from build123d import *

# Parameters (mm, degrees)
EXTRUDE_1_DEPTH     = 44
SKETCH_2_OUTSIDE_W  = 114.91
SKETCH_2_OUTSIDE_H  = 31.91
CUT_EXTRUDE_1_DEPTH = 44
SKETCH_3_W          = 83
SKETCH_3_H          = 84.111264856
CUT_EXTRUDE_2_DEPTH = 2
SKETCH_5_W          = 50
SKETCH_5_H          = 50
CUT_EXTRUDE_3_DEPTH = 6
FILLET_1_R          = 40


with BuildPart() as part:
    # Эскиз1 → Бобышка-Вытянуть1 (new body, symmetric)
    with BuildSketch(Plane(origin=(0, 0, 0), x_dir=(0, 0, -1), z_dir=(1, 0, 0))):
        Polygon((44, 0), (-44, 0), (-44, 3), (-25, 5), (25, 5), (44, 3), align=None)
    extrude(amount=EXTRUDE_1_DEPTH, both=True)

    # Эскиз2 outside → Вырез-Вытянуть1 (cut, symmetric)
    with BuildSketch(Plane.XY):
        with Locations((0, 2.5)):
            Rectangle(SKETCH_2_OUTSIDE_W, SKETCH_2_OUTSIDE_H)
        Polygon((44, 0), (-44, 0), (-44, 3), (-25, 5), (25, 5), (44, 3), align=None, mode=Mode.SUBTRACT)
    extrude(amount=CUT_EXTRUDE_1_DEPTH, both=True, mode=Mode.SUBTRACT)

    # Эскиз3 → Вырез-Вытянуть2 (cut)
    with BuildSketch(Plane.XZ):
        Rectangle(SKETCH_3_W, SKETCH_3_H)
    extrude(amount=-CUT_EXTRUDE_2_DEPTH, mode=Mode.SUBTRACT)

    # Эскиз5 → Вырез-Вытянуть3 (cut, through all)
    with BuildSketch(Plane.XZ):
        Rectangle(SKETCH_5_W, SKETCH_5_H)
    extrude(amount=-CUT_EXTRUDE_3_DEPTH, mode=Mode.SUBTRACT)

    # Скругление1
    fillet_1_edges = [part.edges().sort_by_distance(p)[0] for p in [
        (34.5, 4, -34.5),
        (-34.5, 4, -34.5),
        (-34.5, 4, 34.5),
        (34.5, 4, 34.5),
    ]]
    fillet(fillet_1_edges, radius=FILLET_1_R)


solid = part.part
For this review, take the finished solid that the model builds, in its own axes (mm). A direction names the side the tool comes from. Round coordinates to 2 decimals unless told otherwise and drop trailing zeros. Loops run counter-clockwise (first coordinate to the right, second up) from the corner with the lowest first, then second, coordinate; pieces in that order, holes last. Notation, with made-up numbers: (-19, 67) - (-13, 67) arc R30 ccw to (-13, 102) - close; hole circle Ø5 at (-32, 83). An arc over 180 degrees is marked (long way). One line per item, written item: value. Start each with the question number.
Item 1: Take a section at A-A (x = -1). Give the boundary of the cut face in (y, z), plus the area to 3 significant figures.
Item 2: Clearance check with flat-ended pins moving along their axes: pin 1 Ø8 at (x, z) = (-26, -8) entering from -Y; pin 2 Ø12 at (x, z) = (8, -32) entering from +Y. State where each tip first meets the part, or that it passes through.
Item 3: For L1, parallel to Z at x = 22, y = 2.15; L2, parallel to Z at x = -15.5, y = 1.65, list the stretches that pass through material, from the lowest coordinate up.
Item 4: The part is to be moulded in two halves that separate along X. For faces 1 (the flat face through (-44, 2, -1)), 2 (the flat face through (41.5, 1, -1)), 3 (the flat face through (0.56, 3.79, -36.48)), say which applies: +X half, -X half, draft (parallel to the pull), parting line (faces both ways), or undercut.
Item 5: Take a section at B-B (z = -17.5). Give the boundary of the cut face in (x, y), plus the area to 3 significant figures.
Item 6: For faces 4 (the flat face through (27, 2, 1)), 5 (the flat face through (1, 1, 44)), 6 (the flat face through (25, 3, 0)), list the 3-axis set-ups (+Z, -Z, +X, -X, +Y, -Y) from which the entire face can be reached by the end or side of a thin tool; tool diameter is ignored.
Item 7: Take a section at C-C (y = 1.2). Give the boundary of the cut face in (x, z).
Answer below:
1. outline: (0, -44) - (3, -44) - (5, -25) - (2, -25) - (2, -42.06) - (0, -42.06) - close; (0, 42.06) - (2, 42.06) - (2, 25) - (5, 25) - (3, 44) - (0, 44) - close
1. area: 83.8 mm2
2. pin 1: stops at y = 2
2. pin 2: stops at y = 4.89
3. L1: z = -44 to -25, 25 to 44
3. L2: z = -44 to -42.06, 42.06 to 44
4. face 1: -X half
4. face 2: undercut
4. face 3: draft
5. outline: (-44, 0) - (-41.5, 0) - (-41.5, 2) - (-25, 2) - (-25, 5) - (-44, 3) - close; (25, 2) - (41.5, 2) - (41.5, 0) - (44, 0) - (44, 3) - (25, 5) - close
5. area: 86.0 mm2
6. face 4: -Y
6. face 5: +Z, +X, -X, +Y, -Y
6. face 6: +Y, -Y
7. outline: (-44, -44) - (44, -44) - (44, 44) - (-44, 44) - close; hole (-41.5, -42.06) - (41.5, -42.06) - (41.5, 42.06) - (-41.5, 42.06) - close
